Design review of the part built by this model. Coordinates are the model's own, in mm. Give positions to 0.01 mm unless a question says otherwise; leave off trailing zeros. Loops run counter-clockwise (first coordinate to the right, second up) from the corner with the lowest first, then second, coordinate; pieces in that order, holes last. Notation, with made-up numbers: (62, -12.5) -> (101, -12.5) arc R17 ccw to (101, 13.5) -> close; hole circle Ø5 at (65, -28). An arc over 180 degrees is marked (long way). Answer in a Markdown table with one row per item. Add a question column.
(1) For line 1 (Y direction, x = 0, z = 18); line 2 (Y direction, x = 3.5, z = 18); line 3 (X direction, y = -2.5, z = 17), list the stretches that pass through material, from the lowest coordinate up.
(2) For pin 1 (1 mm diameter, centred on y = 3, z = 24.5, fed in from +X); pin 2 (4 mm diameter, centred on x = -4, z = 22.5, fed in from -Y); pin 3 (3 mm diameter, centred on y = -4, z = 23, fed in from -X), all flat-tipped, find the tip position at first contact; note any pin that passes through.
(3) Draft analysis for pull direction Y (two halves, no side actions). For faces 1 (the cylindrical face through (4.006, -1.262, 19.326)), 2 (the cylindrical face through (-1.08, 4.88, 19.33)), 3 (the flat face through (2, -4, 39.2)), state which applies: +Y half, -Y half, draft (parallel to the pull), parting line (faces both ways), or undercut.
(4) Consider section B-B on z = 35.5. Write out the cut boundary in (x, y).
(5) Consider section A-A on x = 0. Write out the cut boundary in (y, z).
Autodesk Fusion 360 part; units mm, degrees
sketch "Esquisse1" plane through (0, 0, 0) normal (0, 0, 1) x (1, 0, 0)
  circle A0 centre (0, 0) radius 5
  circle A1 centre (0, 0) radius 4.2
  dimension "d1" = 10
  dimension "d2" = 8.4
extrude "Extrusion1" add sketch "Esquisse1" along normal blind 39.2
chamfer "Chanfrein1" distance 0.2 angle 45 1 edges at (-4.6616, -1.8081, 39.2)
chamfer "Chanfrein2" distance 0.2 angle 45 1 edges at (-4.6616, -1.8081, 0)
Values follow:
| question | item | result |
|---|---|---|
| 1 | line 1 | -5 to -4.2, 4.2 to 5 |
| 1 | line 2 | -3.57 to -2.32, 2.32 to 3.57 |
| 1 | line 3 | -4.33 to -3.37, 3.37 to 4.33 |
| 2 | pin 1 | x = 4.33 |
| 2 | pin 2 | y = -4.58 |
| 2 | pin 3 | x = -4.33 |
| 3 | face 1 | undercut |
| 3 | face 2 | parting line |
| 3 | face 3 | draft |
| 4 | outline | circle Ø10 at (0, 0); hole circle Ø8.4 at (0, 0) |
| 5 | outline | (-5, 0.2) -> (-4.8, 0) -> (-4.2, 0) -> (-4.2, 39.2) -> (-4.8, 39.2) -> (-5, 39) -> close; (4.2, 0) -> (4.8, 0) -> (5, 0.2) -> (5, 39) -> (4.8, 39.2) -> (4.2, 39.2) -> close |
